from build123d import *
from OCP.BRepFilletAPI import BRepFilletAPI_MakeChamfer
from build123d.topology import SkipClean

# Parameters (mm, degrees)
SKETCH_1_R      = 2
SKETCH_1_R_2    = 2.7
EXTRUDE_1_DEPTH = 2.5
EXTRUDE_START   = -6.5
SKETCH_1_3_R    = 4.25
SKETCH_1_3_R_2  = 2.7
EXTRUDE_2_DEPTH = 6.5
CHAMFER_1_SIZE  = 2.3
CHAMFER_1_SIZE2 = 1.5
CHAMFER_2_SIZE  = 1.5
CHAMFER_2_SIZE2 = 2.3


with BuildPart() as part:
    # Sketch 1 → Extrude 1 (new body)
    with BuildSketch(Plane.XY):
        with BuildLine():
            ThreePointArc((-16.75, 33.05), (-19.75520382, 31.80520382), (-21, 28.8))
            Line((-21, 28.8), (-21, -28.8))
            ThreePointArc((-21, -28.8), (-19.75520382, -31.80520382), (-16.75, -33.05))
            Line((-16.75, -33.05), (16.75, -33.05))
            ThreePointArc((16.75, -33.05), (19.75520382, -31.80520382), (21, -28.8))
            Line((21, -28.8), (21, 28.8))
            ThreePointArc((21, 28.8), (19.75520382, 31.80520382), (16.75, 33.05))
            Line((16.75, 33.05), (-16.75, 33.05))
        make_face()
        with Locations((-12, 12)):
            Circle(SKETCH_1_R, mode=Mode.SUBTRACT)
        with Locations((-12, -12)):
            Circle(SKETCH_1_R, mode=Mode.SUBTRACT)
        with Locations((-16.75, 28.8)):
            Circle(SKETCH_1_R_2, mode=Mode.SUBTRACT)
        with Locations((-16.75, -28.8)):
            Circle(SKETCH_1_R_2, mode=Mode.SUBTRACT)
        with Locations((12, 12)):
            Circle(SKETCH_1_R, mode=Mode.SUBTRACT)
        with Locations((16.75, 28.8)):
            Circle(SKETCH_1_R_2, mode=Mode.SUBTRACT)
        with Locations((12, -12)):
            Circle(SKETCH_1_R, mode=Mode.SUBTRACT)
        with Locations((16.75, -28.8)):
            Circle(SKETCH_1_R_2, mode=Mode.SUBTRACT)
        Circle(SKETCH_1_R, mode=Mode.SUBTRACT)
    extrude(amount=EXTRUDE_1_DEPTH)

    # Sketch 1_3 → Extrude 2 (add)
    # profile 1 of 4: a face of its own
    with SkipClean():  # the faces are left unmerged after this step: merging them gives an invalid solid
        with BuildSketch(Plane.XY.offset(EXTRUDE_START)):
            with Locations(Location((-16.75, 28.8, 0), (0, 0, 180))):
                Circle(SKETCH_1_3_R)
            with Locations((-16.75, 28.8)):
                Circle(SKETCH_1_3_R_2, mode=Mode.SUBTRACT)
        # profile 2 of 4: a face of its own
        with BuildSketch(Plane.XY.offset(EXTRUDE_START)):
            with Locations(Location((-16.75, -28.8, 0), (0, 0, 180))):
                Circle(SKETCH_1_3_R)
            with Locations((-16.75, -28.8)):
                Circle(SKETCH_1_3_R_2, mode=Mode.SUBTRACT)
        # profile 3 of 4: a face of its own
        with BuildSketch(Plane.XY.offset(EXTRUDE_START)):
            with Locations((16.75, -28.8)):
                Circle(SKETCH_1_3_R)
            with Locations((16.75, -28.8)):
                Circle(SKETCH_1_3_R_2, mode=Mode.SUBTRACT)
        # profile 4 of 4: a face of its own
        with BuildSketch(Plane.XY.offset(EXTRUDE_START)):
            with Locations((16.75, 28.8)):
                Circle(SKETCH_1_3_R)
            with Locations((16.75, 28.8)):
                Circle(SKETCH_1_3_R_2, mode=Mode.SUBTRACT)
        extrude(amount=EXTRUDE_2_DEPTH)

    # Chamfer 1
    chamfer_1_edges = [part.edges().sort_by_distance(p)[0] for p in [
        (-14, 12, 0),
        (10, -12, 0),
    ]]
    chamfer_1_side = [part.faces().sort_by_distance(p)[0] for p in [
        (0, 32.266851866, 0),
    ]]
    chamfer(chamfer_1_edges, length=CHAMFER_1_SIZE, length2=CHAMFER_1_SIZE2, reference=chamfer_1_side[0])

    # Chamfer 2: one chamfer whose edges measure the first distance from different faces: ONE call of the kernel's chamfer builder (chamfer() names one face for all edges)
    chamfer_2_edges_1 = [part.edges().sort_by_distance(p)[0] for p in [
        (-2, 0, 0),
    ]]
    chamfer_2_side_1 = [part.faces().sort_by_distance(p)[0] for p in [
        (-2, 0, 1.25),
    ]]
    chamfer_2_edges_2 = [part.edges().sort_by_distance(p)[0] for p in [
        (-14, -12, 0),
    ]]
    chamfer_2_side_2 = [part.faces().sort_by_distance(p)[0] for p in [
        (-14, -12, 1.25),
    ]]
    chamfer_2_edges_3 = [part.edges().sort_by_distance(p)[0] for p in [
        (10, 12, 0),
    ]]
    chamfer_2_side_3 = [part.faces().sort_by_distance(p)[0] for p in [
        (10, 12, 1.25),
    ]]
    chamfer_2 = BRepFilletAPI_MakeChamfer(part.part.solid().wrapped)
    for e in chamfer_2_edges_1:
        chamfer_2.Add(CHAMFER_2_SIZE, CHAMFER_2_SIZE2, e.wrapped, chamfer_2_side_1[0].wrapped)  # the first distance lies on this face
    for e in chamfer_2_edges_2:
        chamfer_2.Add(CHAMFER_2_SIZE, CHAMFER_2_SIZE2, e.wrapped, chamfer_2_side_2[0].wrapped)  # the first distance lies on this face
    for e in chamfer_2_edges_3:
        chamfer_2.Add(CHAMFER_2_SIZE, CHAMFER_2_SIZE2, e.wrapped, chamfer_2_side_3[0].wrapped)  # the first distance lies on this face
    add(Compound.cast(chamfer_2.Shape()), mode=Mode.REPLACE)


solid = part.part
Check sheet for the modelled part. Datum: model origin and axes. Units: mm. A direction names the side the tool comes from. Round coordinates to 2 decimals unless told otherwise and drop trailing zeros. Order: outer loops, then holes, each group sorted by start corner. A loop starts at its lowest first (then second) coordinate and runs counter-clockwise, first axis right, second up.
(1) Cross-section at A-A, the plane y = 0. Enter the section's corners in (x, z), and give its area (4 significant figures).
(2) Cross-section at D-D, the plane y = 12. Enter the section's corners in (x, z), and give its area (3 significant figures).
(3) Access from +Z, -Z, +X, -X, +Y, -Y to the whole of each face (thin tool, end or side, straight path). Record for faces 1 (the flat face through (-5, 0, 0)), 2 (the cylindrical face through (-13.474, -10.648, 1.993)).
(4) Scan lines: probe 1 along Y at (x, z) = (-12, 1.8); probe 2 along Y at (x, z) = (17.5, -1.5); probe 3 along Z at (x, y) = (4, -19.5). Record each from-to range of solid material in increasing order.
(5) Go/stop test with flat-tipped pins: P1, Ø4, axis at x = 2.5, y = 0, coming from the -Z side; P2, Ø6.5, axis at x = -12, y = 12, coming from the -Z side; P3, Ø5, axis at x = -12, y = -12, coming from the -Z side; P4, Ø5, axis at x = 16.75, y = 28.8, coming from the -Z side. Record where each tip stops, or that it passes through.
(6) Cross-section at B-B, the plane z = -4.75. Enter the section's corners in (x, y), and give its area (3 significant figures).
(7) Draft check along Y on faces 3 (the flat face through (0, 33.05, 1)), 4 (the flat face through (21, 0, 1)), 5 (the conical face through (-0.46, -2.09, 1.41)). Enter one of: pulls with the +Y half, pulls with the -Y half, needs draft (parallel to the pull), parting line crosses it, or undercut.
(8) Cross-section at C-C, the plane x = 0. Enter the section's corners in (y, z), and give its area (3 significant figures).
Check sheet entries:
1. outline: (-21, 0) - (-4.3, 0) - (-2, 1.5) - (-2, 2.5) - (-21, 2.5) - close; (2, 1.5) - (4.3, 0) - (21, 0) - (21, 2.5) - (2, 2.5) - close
1. area: 91.55 mm2
2. outline: (-21, 0) - (-16.3, 0) - (-14, 1.5) - (-14, 2.5) - (-21, 2.5) - close; (-10, 1.5) - (-7.7, 0) - (7.7, 0) - (10, 1.5) - (10, 2.5) - (-10, 2.5) - close; (14, 1.5) - (16.3, 0) - (21, 0) - (21, 2.5) - (14, 2.5) - close
2. area: 78.1 mm2
3. face 1: -Z
3. face 2: +Z, -Z
4. probe 1: y = -33.05 to -14, -10 to 10, 14 to 33.05
4. probe 2: y = -32.98 to -31.39, -26.21 to -24.62, 24.62 to 26.21, 31.39 to 32.98
4. probe 3: z = 0 to 2.5
5. P1: stops at z = 0
5. P2: stops at z = 0.68
5. P3: stops at z = 1.17
5. P4: passes through
6. outline: circle Ø8.5 at (-16.75, -28.8); circle Ø8.5 at (-16.75, 28.8); circle Ø8.5 at (16.75, -28.8); circle Ø8.5 at (16.75, 28.8); hole circle Ø5.4 at (-16.75, -28.8); hole circle Ø5.4 at (-16.75, 28.8); hole circle Ø5.4 at (16.75, -28.8); hole circle Ø5.4 at (16.75, 28.8)
6. area: 135 mm2
7. face 3: pulls with the +Y half
7. face 4: needs draft
7. face 5: undercut
8. outline: (-33.05, 0) - (-4.3, 0) - (-2, 1.5) - (-2, 2.5) - (-33.05, 2.5) - close; (2, 1.5) - (4.3, 0) - (33.05, 0) - (33.05, 2.5) - (2, 2.5) - close
8. area: 152 mm2
